Check sheet for the modelled part. Datum: model origin and axes. Units: mm. A direction names the side the tool comes from. Give positions to 0.01 mm unless a question says otherwise; leave off trailing zeros. Loops run counter-clockwise (first coordinate to the right, second up) from the corner with the lowest first, then second, coordinate; pieces in that order, holes last. Notation, with made-up numbers: M 54.25,-19.75 L 110.25,-19.75 A24 cw 110.25,10.25 Z; hole C 76,45.25 d8. An arc over 180 degrees is marked long. Use one line per item in the form item = value.
Autodesk Inventor part; units mm, degrees
ref_plane "dia1_XY" through (0, 3.175, 0) normal (1, 0, 0) x (0, 0, -1)
ref_plane "dia1_YZ" through (0, 3.175, 0) normal (0, 0, -1) x (0, 1, 0)
ref_plane "dia1_ZX" through (0, 3.175, 0) normal (0, 1, 0) x (1, 0, 0)
sketch "Sketch_1" plane through (0, 0, 0) normal (0, 0, 1) x (1, 0, 0)
  line L0 (201.93, 0) -> (0, 0)
  line L1 (0, 0) -> (0, 3.175)
  line L2 (0, 3.175) -> (129.3876, 3.175)
  line L3 (129.3876, 3.175) -> (129.3876, 9.6202)
  line L4 (129.3876, 9.6202) -> (201.93, 9.6202)
  line L5 (201.93, 9.6202) -> (201.93, 0)
  line L6 (201.93, 0) -> (0, 0)
revolve "Revolution1" add sketch "Sketch_1" angle 360 about axis through (201.93, 0, 0) along (1, 0, 0)
sketch "Sketch_3" plane through (0, 0, 0) normal (0, 0, 1) x (1, 0, 0)
  line L0 (0, 0) -> (-12.7, 0)
  line L1 (-12.7, 0) -> (-12.7, 2.634)
  line L2 (-12.7, 2.634) -> (-12.159, 3.175)
  line L3 (-12.159, 3.175) -> (0, 3.175)
  line L4 (0, 3.175) -> (0, 0)
  line L5 (0, 0) -> (-12.7, 0)
revolve "Revolution2" add sketch "Sketch_3" angle 360 about axis through (0, 0, 0) along (1, 0, 0)
sketch "Sketch_30" plane through (0, 0, 0) normal (0, 0, 1) x (1, 0, 0)
  line L0 (0, 0) -> (-0.254, 0)
  line L1 (-0.254, 2.921) -> (0, 2.921)
  line L2 (0, 2.921) -> (0, 3.429)
  line L3 (0, 3.429) -> (-0.254, 3.429)
  line L4 (-0.254, 3.429) -> (-0.254, 2.921)
revolve "Revolution3" cut sketch "Sketch_30" angle 360 about axis through (0, 0, 0) along (1, 0, 0)
ref_plane "dia1_XY" through (0, 3.175, 0) normal (1, 0, 0) x (0, 0, -1)
ref_plane "dia1_YZ" through (0, 3.175, 0) normal (0, 0, -1) x (0, 1, 0)
ref_plane "dia1_ZX" through (0, 3.175, 0) normal (0, 1, 0) x (1, 0, 0)
ref_plane "dia12_XY" through (0, 0, 10.9537) normal (1, 0, 0) x (0, 0, -1)
ref_plane "dia12_YZ" through (0, 0, 10.9537) normal (0, 0, -1) x (0, 1, 0)
ref_plane "dia12_ZX" through (0, 0, 10.9537) normal (0, 1, 0) x (1, 0, 0)
ref_plane "dia1r_XY" through (0, 0, 10.2235) normal (1, 0, 0) x (0, 0, -1)
ref_plane "dia1r_YZ" through (0, 0, 10.2235) normal (0, 0, -1) x (0, 1, 0)
ref_plane "dia1r_ZX" through (0, 0, 10.2235) normal (0, 1, 0) x (1, 0, 0)
ref_plane "dia2_XY" through (0, -3.175, 0) normal (1, 0, 0) x (0, 0, -1)
ref_plane "dia2_YZ" through (0, -3.175, 0) normal (0, 0, -1) x (0, 1, 0)
ref_plane "dia2_ZX" through (0, -3.175, 0) normal (0, 1, 0) x (1, 0, 0)
ref_plane "dia22_XY" through (0, 0, -10.9537) normal (1, 0, 0) x (0, 0, -1)
ref_plane "dia22_YZ" through (0, 0, -10.9537) normal (0, 0, -1) x (0, 1, 0)
ref_plane "dia22_ZX" through (0, 0, -10.9537) normal (0, 1, 0) x (1, 0, 0)
ref_plane "dia2r_XY" through (0, 0, -10.2235) normal (1, 0, 0) x (0, 0, -1)
ref_plane "dia2r_YZ" through (0, 0, -10.2235) normal (0, 0, -1) x (0, 1, 0)
ref_plane "dia2r_ZX" through (0, 0, -10.2235) normal (0, 1, 0) x (1, 0, 0)
ref_plane "rl1_XY" through (-12.7, 0, 0) normal (1, 0, 0) x (0, 0, -1)
ref_plane "rl1_YZ" through (-12.7, 0, 0) normal (0, 0, -1) x (0, 1, 0)
ref_plane "rl1_ZX" through (-12.7, 0, 0) normal (0, 1, 0) x (1, 0, 0)
ref_plane "rl2_XY" through (0, 0, 0) normal (1, 0, 0) x (0, 0, -1)
ref_plane "rl2_YZ" through (0, 0, 0) normal (0, 0, -1) x (0, 1, 0)
ref_plane "rl2_ZX" through (0, 0, 0) normal (0, 1, 0) x (1, 0, 0)
ref_plane "rod_cp_XY" through (0, 0, 0) normal (1, 0, 0) x (0, 0, -1)
ref_plane "rod_cp_YZ" through (0, 0, 0) normal (0, 0, -1) x (0, 1, 0)
ref_plane "rod_cp_ZX" through (0, 0, 0) normal (0, 1, 0) x (1, 0, 0)
ref_plane "stroke1_XY" through (0, 0, 0) normal (1, 0, 0) x (0, 0, -1)
ref_plane "stroke1_YZ" through (0, 0, 0) normal (0, 0, -1) x (0, 1, 0)
ref_plane "stroke1_ZX" through (0, 0, 0) normal (0, 1, 0) x (1, 0, 0)
ref_plane "thd1_XY" through (-12.7, 3.175, 0) normal (1, 0, 0) x (0, 0, -1)
ref_plane "thd1_YZ" through (-12.7, 3.175, 0) normal (0, 0, -1) x (0, 1, 0)
ref_plane "thd1_ZX" through (-12.7, 3.175, 0) normal (0, 1, 0) x (1, 0, 0)
ref_plane "thd2_XY" through (-12.7, -3.175, 0) normal (1, 0, 0) x (0, 0, -1)
ref_plane "thd2_YZ" through (-12.7, -3.175, 0) normal (0, 0, -1) x (0, 1, 0)
ref_plane "thd2_ZX" through (-12.7, -3.175, 0) normal (0, 1, 0) x (1, 0, 0)
ref_plane "to_rod_clevis_XY" through (-16.764, 0, 0) normal (1, 0, 0) x (0, 0, -1)
ref_plane "to_rod_clevis_YZ" through (-16.764, 0, 0) normal (0, 0, -1) x (0, 1, 0)
ref_plane "to_rod_clevis_ZX" through (-16.764, 0, 0) normal (0, 1, 0) x (1, 0, 0)
properties part number "C-043.5-HRP0000_rod"
1) Section check A-A (z = 0). Record the cut outline in (x, y) (3 decimals).
Evaluation:
outline = M -12.7,-2.634 L -12.159,-3.175 L -0.254,-3.175 L -0.254,-2.921 L 0,-2.921 L 0,-3.175 L 129.388,-3.175 L 129.388,-9.62 L 201.93,-9.62 L 201.93,9.62 L 129.388,9.62 L 129.388,3.175 L 0,3.175 L 0,2.921 L -0.254,2.921 L -0.254,3.175 L -12.159,3.175 L -12.7,2.634 Z
2) Section check C-C (x = 18). Record the cut outline in (y, z) (3 decimals), then the cut area to 3 significant figures.
Evaluation:
outline = C 0,0 d6.35
area = 31.7 mm^2
3) Section check D-D (x = 138). Record the cut outline in (y, z).
Evaluation:
outline = C 0,0 d19.24
4) Depth check by flat-ended pin: pin 1 Ø1 at (y, z) = (2.5, 6) entering from -X; pin 2 Ø10 at (x, z) = (117.5, -5.5) entering from +Y; pin 3 Ø5 at (x, z) = (87.5, -3.5) entering from -Y. Enter the tip coordinate at first touch or a pass-through.
Evaluation:
pin_1 = 129.39
pin_2 = 3.14
pin_3 = -3.01
5) Scan lines: line 1 (X direction, y = -3.25, z = -7); line 2 (Y direction, x = 108, z = 0.25); line 3 (Z direction, x = 44, y = 1.25). Record each from-to range of solid material in increasing order.
Evaluation:
line_1 = 129.39 to 201.93
line_2 = -3.17 to 3.17
line_3 = -2.92 to 2.92
6) Set-up check for faces 1 (the face through (65.6, -0.69, -3.1)), 2 (the face through (-12.7, 0, 0)): record each of +Z, -Z, +X, -X, +Y, -Y from which the full face is reachable in a straight line by a thin tool's end or side.
Evaluation:
face_1 = -X
face_2 = +Z, -Z, -X, +Y, -Y
